```python
from build123d import *

# Parameters (mm, degrees)
F0_W     = 31
F0_H     = 30
F1_DEPTH = 28.55
F2_R     = 1.15
F3_DEPTH = 57.101
F4_R     = 4.175
F5_DEPTH = 5.5
F7_DEPTH = 1
F8_R     = 6


with BuildPart() as f1:
    # F0 (on Front) → F1 (new body, symmetric)
    with BuildSketch(Plane.XZ):
        Rectangle(F0_W, F0_H)
    extrude(amount=F1_DEPTH, both=True)

    # F2 (on face) → F3 (cut, through all)
    with BuildSketch(Plane(origin=(0, 28.55, 0), x_dir=(-1, 0, 0), z_dir=(0, 1, 0))):
        with Locations((-2.85, 2.85)):
            Circle(F2_R)
        with Locations((2.85, 2.85)):
            Circle(F2_R)
        with Locations((-2.85, -2.85)):
            Circle(F2_R)
        with Locations((2.85, -2.85)):
            Circle(F2_R)
    extrude(amount=-F3_DEPTH, mode=Mode.SUBTRACT)

    # F4 (on face) → F5 (join)
    with BuildSketch(Plane.XZ.offset(28.55)):
        with Locations((6.725, 7.965)):
            Circle(F4_R)
        with Locations((-6.725, 7.965)):
            Circle(F4_R)
    extrude(amount=F5_DEPTH)

    # F6 (on face) → F7 (join)
    with BuildSketch(Plane.XZ.offset(34.05)):
        with BuildLine():
            add(Edge.make_bspline(
                [(13.5, 8), (13.5, 19.691343), (-6.75, 13.845671), (-27, 8), (-6.75, 2.154329), (13.5, -3.691343), (13.5, 8)],
                knots=[0, 0, 0, 2.094395, 2.094395, 4.18879, 4.18879, 6.283185, 6.283185, 6.283185], degree=2, weights=[1, 0.5, 1, 0.5, 1, 0.5, 1]))
        make_face()
    extrude(amount=F7_DEPTH)

    # F8
    f8_edges = [f1.edges().sort_by_distance(p)[0] for p in [
        (-15.5, 0, 15),
        (15.5, 0, 15),
        (-15.5, 0, -15),
        (15.5, 0, -15),
    ]]
    fillet(f8_edges, radius=F8_R)


solid = f1.part
```
Could you check a few things on this model? Use its own coordinates, in mm. A direction names the side the tool comes from. Round coordinates to 2 decimals unless told otherwise and drop trailing zeros. Write each loop counter-clockwise with the first axis right and the second up, starting at its lowest first coordinate (ties: lowest second). Pieces come first, ordered by that corner, then holes.
(1) Suppose I cut it at B-B on y = 17.5. Write out the boundary of the cut face in (x, z).
Findings below:
outline: (-15.5, -9) arc R6 ccw to (-9.5, -15) - (9.5, -15) arc R6 ccw to (15.5, -9) - (15.5, 9) arc R6 ccw to (9.5, 15) - (-9.5, 15) arc R6 ccw to (-15.5, 9) - close; hole circle Ø2.3 at (-2.85, -2.85); hole circle Ø2.3 at (-2.85, 2.85); hole circle Ø2.3 at (2.85, -2.85); hole circle Ø2.3 at (2.85, 2.85)
(2) If I drill on probe 1 along Z at (x, y) = (2.85, 14); probe 2 along Z at (x, y) = (2, -13); probe 3 along Y at (x, z) = (-7, 3.5), over which ranges is the centre line in solid material (lowest first)?
Findings below:
probe 1: z = -15 to -4, -1.7 to 1.7, 4 to 15
probe 2: z = -15 to -3.62, -2.08 to 2.08, 3.62 to 15
probe 3: y = -35.05 to -34.05, -28.55 to 28.55
(3) Thinking about a two-plate mould opening in Y: for faces 4 (the face through (-1, -35.05, 9)), 5 (the face through (0, 0, 15)), 6 (the face through (-10.896, -31.262, 8.149)), which applies, +Y half, -Y half, draft (parallel to the pull), parting line (faces both ways), or undercut?
Findings below:
face 4: -Y half
face 5: draft
face 6: undercut
(4) Which directions (+Z, -Z, +X, -X, +Y, -Y) give clear straight access to the entire face, cutting with the end or side of a thin tool? Please do faces 1 (the face through (-1, -34.05, 8)), 2 (the face through (-13.789, 0.4, 13.196)), 3 (the face through (4, 0.4, 2.9)).
Findings below:
face 1: none
face 2: +Z, -X, +Y, -Y
face 3: +Y
(5) For pin 1 (1.4 mm diameter, centred on x = 2.85, z = 2.85, fed in from +Y); pin 2 (3.5 mm diameter, centred on x = 2.85, z = -2.85, fed in from -Y); pin 3 (2 mm diameter, centred on x = -2.85, z = -2.85, fed in from +Y), each with a flat end and sliding along its axis, tell me the tip position at first contact or that it passes through.
Findings below:
pin 1: stops at y = -34.05
pin 2: stops at y = -28.55
pin 3: passes through
(6) Suppose I cut it at C-C on z = 2.85. State how many separate pieces and enclosed holes the cut face has, and give its area (3 significant figures).
Findings below:
separate pieces: 4
enclosed holes: 0
area: 1,520 mm2
(7) Suppose I cut it at A-A on z = -2.85. Write out the boundary of the cut face in (x, y), and give its area (3 significant figures).
Findings below:
outline: (-15.5, -28.55) - (-4, -28.55) - (-4, 28.55) - (-15.5, 28.55) - close; (-1.7, -28.55) - (1.7, -28.55) - (1.7, 28.55) - (-1.7, 28.55) - close; (4, -28.55) - (15.5, -28.55) - (15.5, 28.55) - (4, 28.55) - close
area: 1,510 mm2
